Read the model definition and answer for the solid it produces. Units are mm, in the model's axes. Face numbers are marked on the shaded views. A direction names the side the tool comes from. Round coordinates to 2 decimals unless told otherwise and drop trailing zeros. Loops run counter-clockwise (first coordinate to the right, second up) from the corner with the lowest first, then second, coordinate; pieces in that order, holes last. Notation, with made-up numbers: (62, 87.25) - (68, 87.25) arc R22 cw to (68, 96.25) - close; hole circle Ø5 at (56.5, 86.5). An arc over 180 degrees is marked (long way). Answer as CSV lines item,"result".
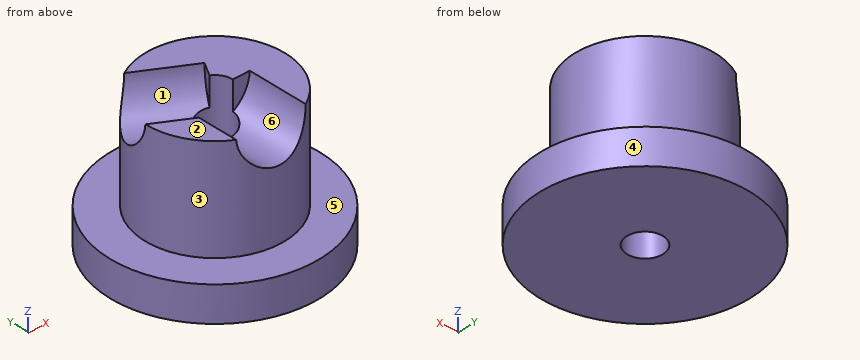
Autodesk Fusion 360 part; units mm, degrees
sketch "Sketch1" plane through (0, 0, 0) normal (0, 0, 1) x (1, 0, 0)
  circle A0 centre (0, 0) radius 6.35
  circle A1 centre (0, 0) radius 9.525
  dimension "d1" = 12.7
  dimension "d24" = 19.05
extrude "Extrude1" add sketch "Sketch1" along normal blind 12.7 contours A0
ref_plane "WorkPlane1" through (0, -6.35, 16.0163) normal (0, -1, 0) x (-1, 0, 0)
sketch "Sketch2" plane through (0, -6.35, 16.0163) normal (0, -1, 0) x (1, 0, 0)
  line L0 (6.35, -3.3163) -> (-6.35, -3.3163)
  line L1 (6.35, -16.0163) -> (-6.35, -16.0163)
  point P0 (0, -3.3163)
ref_plane "WorkPlane2" through (0, 0, 9.525) normal (0, 0, 1) x (1, 0, 0)
sketch "Sketch4" plane through (0, 0, 9.525) normal (0, 0, 1) x (1, 0, 0)
  circle A0 centre (0, 0) radius 6.35
  line L0 (0, 0) -> (0, -6.35) construction
  line L1 (0, 0) -> (5.4993, 3.175) construction
  line L2 (0, 0) -> (-5.4993, 3.175) construction
  dimension "d22" = 360
hole "Hole1" at (0, -6.35, 12.7) direction (0, 1, 0) diameter 6.35 depth 6.35 tip angle 180
pattern_circular "C-Pattern1" count 3 over 360 about axis through (0, 0, 0) along (0, 0, 1) of "Hole1"
extrude "Extrude2" cut sketch "Sketch4" against normal blind 0.127 from surface at 3.175
hole "Hole2" at (0, 0, 0) direction (0, 0, 1) diameter 3.2639 depth 12.573 tip angle 180
extrude "Extrude3" add sketch "Sketch1" along normal blind 3.175
equation "d5 = d1 / 2"
1) A cutting plane is placed at A-A, the plane z = 10.5. Determine the outline of the cut face in (x, y).
Entries:
outline,"(-6.27, 0.98) arc R6.35 ccw to (-2.29, -5.92) - (-2.29, -1.32) - close; (-3.98, 4.94) - (1.14, 1.98) - (0.82, 1.41) arc R1.63 cw to (1.63, 0) - (2.29, 0) - (2.29, -5.92) arc R6.35 ccw (long way) to start"
2) A tool of negligible diameter and unlimited length cuts with its end or side. For the marked faces 4, 5 and 6, from which of +Z, -Z, +X, -X, +Y, -Y can it reach the whole face along a straight path? Write none if from no direction.
Entries:
face 4,"+Z, -Z"
face 5,"+Z"
face 6,"+Z, -Y"
3) Each of these flat-tipped pins is pushed along its axis until it touches: P1, Ø1, axis at x = -3.5, z = 6, coming from the +Y side; P2, Ø1.7, axis at x = 2.5, z = 11.5, coming from the -Y side; P3, Ø5, axis at x = -5, z = 4, coming from the -Y side. Where does it stop, or does it pass through?
Entries:
P1,"stops at y = 5.6"
P2,"stops at y = -5.87"
P3,"stops at y = -9.15"
4) A cutting plane is placed at D-D, the plane x = 3.5. Determine the outline of the cut face in (y, z) (3 decimals), plus the area to 3 significant figures.
Entries:
outline,"(-8.859, 0) - (8.859, 0) - (8.859, 3.175) - (5.298, 3.175) - (5.298, 12.573) - (-5.298, 12.573) - (-5.298, 3.175) - (-8.859, 3.175) - close"
area,"156 mm^2"
5) Find the intervals of material crossed by line 1 (X direction, y = 0, z = 4.75); line 2 (Y direction, x = 0, z = 3) (3 decimals), in increasing order.
Entries:
line 1,"x = -6.35 to -1.63, 1.63 to 6.35"
line 2,"y = -9.525 to -1.632, 1.632 to 9.525"
6) The mould has two halves that part along X. Classify the marked faces 1, 2 and 3: pulls with the +X half, pulls with the -X half, needs draft (parallel to the pull), parting line crosses it, or undercut.
Entries:
face 1,"undercut"
face 2,"needs draft"
face 3,"parting line crosses it"
7) A cutting plane is placed at C-C, the plane y = 5.75. Determine the outline of the cut face in (x, z) (3 decimals).
Entries:
outline,"(-7.594, 0) - (7.594, 0) - (7.594, 3.175) - (2.694, 3.175) - (2.694, 12.573) - (-2.694, 12.573) - (-2.694, 3.175) - (-7.594, 3.175) - close"
8) A cutting plane is placed at B-B, the plane z = 4.25. Determine the outline of the cut face in (x, y), plus the area to 3 significant figures.
Entries:
outline,"circle Ø12.7 at (0, 0); hole circle Ø3.26 at (0, 0)"
area,"118 mm^2"
